The listing builds one solid part. Answer for the finished solid, in the listing's coordinates (mm). Face numbers are marked on the shaded views. A direction names the side the tool comes from. Give positions to 0.01 mm unless a question says otherwise; leave off trailing zeros. Order: outer loops, then holes, each group sorted by start corner. A loop starts at its lowest first (then second) coordinate and runs counter-clockwise, first axis right, second up. Notation, with made-up numbers: (34, 13.25) -> (74, 13.25) arc R16 cw to (74, 42.25) -> close; hole circle Ø9 at (78, 34.25). An arc over 180 degrees is marked (long way). Answer as a JSON object with one key per item and string values. Group by question number.
```python
from build123d import *

# Parameters (mm, degrees)
F1_DEPTH = 35.9918
F2_W     = 24.003
F2_H     = 16.9418
F3_DEPTH = 20.8534
F4_W     = 24.9682
F4_H     = 8.9916
F5_DEPTH = 24.9428


with BuildPart() as f1:
    # F0 (on Top) → F1 (new body)
    with BuildSketch(Plane.XY):
        Polygon((0, 35.9918), (0, 0), (56.007, 0), (56.007, 35.9918), (40.004998, 35.9918), (40.004998, 24.053801), (16.001999, 24.053801), (16.001999, 35.9918), align=None)
    extrude(amount=-F1_DEPTH)

    # F2 (on face) → F3 (cut)
    with BuildSketch(Plane.YZ.offset(56.007)):
        with Locations((12.0015, -27.5209)):
            Rectangle(F2_W, F2_H)
    extrude(amount=-F3_DEPTH, mode=Mode.SUBTRACT)

    # F4 (on face) → F5 (cut)
    with BuildSketch(Plane.XY):
        with Locations((12.4841, 4.4958)):
            Rectangle(F4_W, F4_H)
    extrude(amount=-F5_DEPTH, mode=Mode.SUBTRACT)


solid = f1.part
```
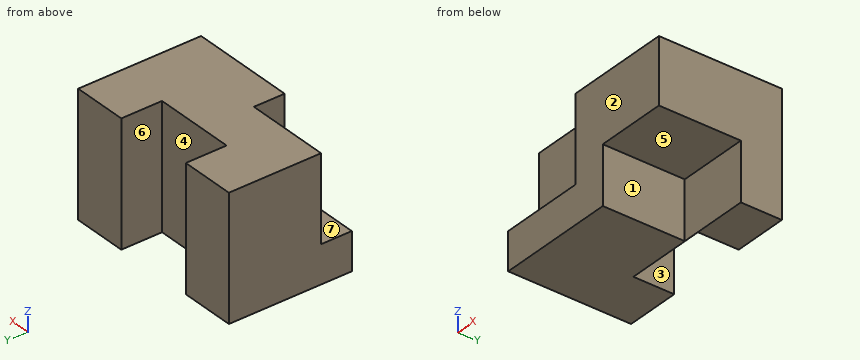
(1) A cutting plane is placed at C-C (z = -29). Determine the outline of the cut face in (x, y) (3 decimals).
(2) A cutting plane is placed at A-A (y = 26). Determine the outline of the cut face in (x, z) (3 decimals).
(3) For a pull along X with two mould halves and no side action, classify the marked faces 1, 2, 3 and 4 as +X half, -X half, draft (parallel to the pull), parting line (faces both ways), or undercut.
(4) Find the intervals of material crossed by line 1 along X through (y, z) = (25.5, -12) (3 decimals); line 2 along Y through (x, z) = (34, -16); line 3 along Z through (x, y) = (45, 22), in increasing order. Write a range as [from, to].
(5) Which of the six approach directions +Z, -Z, +X, -X, +Y, -Y give full straight-line access (tool end or side, diameter ignored) to the marked faces 5, 6 and 7?
(6) A cutting plane is placed at D-D (y = 5). Determine the outline of the cut face in (x, z).
(7) A cutting plane is placed at B-B (x = 22). Determine the outline of the cut face in (y, z), and give its area (3 significant figures).
(8) Flat-ended cylindrical pins translate along their axes: pin 1 Ø7.5 at (x, z) = (10.5, -8) entering from -Y; pin 2 Ø12 at (x, z) = (29, -9) entering from +Y; pin 3 Ø10 at (x, y) = (47, 5.5) entering from -Z. Find the tip coordinate at first contact, or state that the pin passes through.
Check sheet entries:
{
 "1": {"outline": "(0, 0) -> (35.154, 0) -> (35.154, 24.003) -> (56.007, 24.003) -> (56.007, 35.992) -> (40.005, 35.992) -> (40.005, 24.054) -> (16.002, 24.054) -> (16.002, 35.992) -> (0, 35.992) -> close"},
 "2": {"outline": "(0, -35.992) -> (16.002, -35.992) -> (16.002, 0) -> (0, 0) -> close; (40.005, -35.992) -> (56.007, -35.992) -> (56.007, 0) -> (40.005, 0) -> close"},
 "3": {"face 1": "+X half", "face 2": "draft", "face 3": "undercut", "face 4": "undercut"},
 "4": {"line 1": "x = [0, 16.002], [40.005, 56.007]", "line 2": "y = [0, 24.05]", "line 3": "z = [-19.05, 0]"},
 "5": {"face 5": "-Z, +X, -Y", "face 6": "+Z, -Z, +Y", "face 7": "+Z, -X, -Y"},
 "6": {"outline": "(0, -35.99) -> (35.15, -35.99) -> (35.15, -19.05) -> (56.01, -19.05) -> (56.01, 0) -> (24.97, 0) -> (24.97, -24.94) -> (0, -24.94) -> close"},
 "7": {"outline": "(0, -35.99) -> (24.05, -35.99) -> (24.05, 0) -> (8.99, 0) -> (8.99, -24.94) -> (0, -24.94) -> close", "area": "641 mm2"},
 "8": {"pin 1": "stops at y = 8.99", "pin 2": "stops at y = 24.05", "pin 3": "stops at z = -19.05"}
}
